from build123d import *

# Parameters (mm, degrees)
SKETCH1_R           = 30
SKETCH1_R_2         = 2
BOSS_EXTRUDE1_DEPTH = 1.5
CUT_EXTRUDE1_DEPTH  = 10


with BuildPart() as part:
    # Sketch1 → Boss-Extrude1 (new body)
    with BuildSketch(Plane.XY):
        Circle(SKETCH1_R)
        with Locations((15, 0)):
            Circle(SKETCH1_R_2, mode=Mode.SUBTRACT)
        with Locations((-15, 0)):
            Circle(SKETCH1_R_2, mode=Mode.SUBTRACT)
    extrude(amount=BOSS_EXTRUDE1_DEPTH)

    # Sketch2 → Cut-Extrude1 (cut)
    with BuildSketch(Plane(origin=(0, 0, 0), x_dir=(-1, 0, 0), z_dir=(0, 0, -1))):
        with BuildLine():
            Line((7.071067812, 7.071067812), (9.899494937, 9.899494937))
            ThreePointArc((9.899494937, 9.899494937), (0, 14), (-9.899494937, 9.899494937))
            Line((-9.899494937, 9.899494937), (-7.071067812, 7.071067812))
            ThreePointArc((-7.071067812, 7.071067812), (-10, 0), (-7.071067812, -7.071067812))
            Line((-7.071067812, -7.071067812), (-9.899494937, -9.899494937))
            ThreePointArc((-9.899494937, -9.899494937), (0, -14), (9.899494937, -9.899494937))
            Line((9.899494937, -9.899494937), (7.071067812, -7.071067812))
            ThreePointArc((7.071067812, -7.071067812), (10, 0), (7.071067812, 7.071067812))
        make_face()
    extrude(amount=-CUT_EXTRUDE1_DEPTH, mode=Mode.SUBTRACT)


solid = part.part
The listing builds one solid part. Answer for the finished solid, in the listing's coordinates (mm). A direction names the side the tool comes from. Coordinates: 2 decimals unless noted, no trailing zeros. Order: outer loops, then holes, each group sorted by start corner. A loop starts at its lowest first (then second) coordinate and runs counter-clockwise, first axis right, second up. Notation, with made-up numbers: (8, 78.5) -> (18, 78.5) arc R31 ccw to (18, 110.5) -> close; hole circle Ø4 at (16, 52.25). An arc over 180 degrees is marked (long way). Answer in a Markdown table with one row per item. Add a question column.
Item 1: Find section A-A (x = 0). Write down the section's boundary in (y, z), then the cut area to 3 significant figures.
Item 2: Find section D-D (y = 0). Write down the section's boundary in (x, z).
Item 3: Find section B-B (y = 6). Write down the section's boundary in (x, z), then the cut area to 3 significant figures.
Item 4: Find the intervals of material crossed by L1, parallel to Y at x = -9, z = 1.4; L2, parallel to Y at x = 8.5, z = 0.75; L3, parallel to Y at x = -15, z = 1.05, in increasing order. Write a range as from..to.
Item 5: Which of the six approach directions +Z, -Z, +X, -X, +Y, -Y give full straight-line access (tool end or side, diameter ignored) to faces 4 (the face through (0, -14, 1)), 5 (the face through (13, -6, 0))?
Item 6: Find section C-C (z = 1.25). Write down the section's boundary in (x, y).
Item 7: Determine the mould class of faces 1 (the face through (13, -6, 1.5)), 2 (the face through (10, 0, 1)), 3 (the face through (-29.97, 1.32, 0.74)) for opening direction X: +X half, -X half, draft (parallel to the pull), parting line (faces both ways), or undercut.
Result set:
| question | item | result |
|---|---|---|
| 1 | outline | (-30, 0) -> (-14, 0) -> (-14, 1.5) -> (-30, 1.5) -> close; (14, 0) -> (30, 0) -> (30, 1.5) -> (14, 1.5) -> close |
| 1 | area | 48.0 mm² |
| 2 | outline | (-30, 0) -> (-17, 0) -> (-17, 1.5) -> (-30, 1.5) -> close; (-13, 0) -> (-10, 0) -> (-10, 1.5) -> (-13, 1.5) -> close; (10, 0) -> (13, 0) -> (13, 1.5) -> (10, 1.5) -> close; (17, 0) -> (30, 0) -> (30, 1.5) -> (17, 1.5) -> close |
| 3 | outline | (-29.39, 0) -> (-8, 0) -> (-8, 1.5) -> (-29.39, 1.5) -> close; (8, 0) -> (29.39, 0) -> (29.39, 1.5) -> (8, 1.5) -> close |
| 3 | area | 64.2 mm² |
| 4 | L1 | y = -28.62..-10.72, -9..-4.36, 4.36..9, 10.72..28.62 |
| 4 | L2 | y = -28.77..-11.12, -8.5..-5.27, 5.27..8.5, 11.12..28.77 |
| 4 | L3 | y = -25.98..-2, 2..25.98 |
| 5 | face 4 | +Z, -Z |
| 5 | face 5 | -Z, +X, -X, +Y, -Y |
| 6 | outline | circle Ø60 at (0, 0); hole circle Ø4 at (-15, 0); hole (-9.9, -9.9) arc R14 ccw to (9.9, -9.9) -> (7.07, -7.07) arc R10 ccw to (7.07, 7.07) -> (9.9, 9.9) arc R14 ccw to (-9.9, 9.9) -> (-7.07, 7.07) arc R10 ccw to (-7.07, -7.07) -> close; hole circle Ø4 at (15, 0) |
| 7 | face 1 | draft |
| 7 | face 2 | undercut |
| 7 | face 3 | parting line |
